Could you check a few things on this model? Use its own coordinates, in mm. A direction names the side the tool comes from. Coordinates: 2 decimals unless noted, no trailing zeros. Loops run counter-clockwise (first coordinate to the right, second up) from the corner with the lowest first, then second, coordinate; pieces in that order, holes last. Notation, with made-up numbers: M 64,54 L 120,54 A34 cw 120,90 Z; hole C 81.5,-9 d2. An arc over 180 degrees is marked long. Write each question's results on one line, items separated by ' | '.
Autodesk Fusion 360 part; units mm, degrees
sketch "main" plane through (0, 0, 0) normal (0, 0, 1) x (1, 0, 0)
  line L0 (-50, 15) -> (50, 15)
  line L1 (50, 15) -> (50, -15)
  line L2 (50, -15) -> (-50, -15)
  line L3 (-50, -15) -> (-50, 15)
  line L4 (-50, 15) -> (50, -15) construction
  line L5 (50, 15) -> (-50, -15) construction
  line L6 (30, 15) -> (-30, 15) construction
  line L7 (-30, 15) -> (-30, -15) construction
  line L8 (-30, -15) -> (30, -15) construction
  line L9 (30, -15) -> (30, 15) construction
  line L10 (-50, 15) -> (-30, -15) construction
  line L11 (-30, 15) -> (-50, -15) construction
  circle A0 centre (-40, 0) radius 2.75
  line L12 (30, 15) -> (50, -15) construction
  line L13 (50, 15) -> (30, -15) construction
  circle A1 centre (40, 0) radius 2.75
  line L14 (-50, -15) -> (50, -15)
  line L15 (50, -15) -> (50, -6.5)
  line L16 (50, -6.5) -> (-50, -6.5)
  line L17 (-50, -6.5) -> (-50, -15)
  line L18 (35.95, -4.05) -> (44.05, -4.05)
  line L19 (44.05, -4.05) -> (44.05, 4.05)
  line L20 (44.05, 4.05) -> (35.95, 4.05)
  line L21 (35.95, 4.05) -> (35.95, -4.05)
  line L22 (35.95, -4.05) -> (44.05, 4.05) construction
  line L23 (44.05, -4.05) -> (35.95, 4.05) construction
  line L24 (-44.05, -4.05) -> (-35.95, -4.05)
  line L25 (-35.95, -4.05) -> (-35.95, 4.05)
  line L26 (-35.95, 4.05) -> (-44.05, 4.05)
  line L27 (-44.05, 4.05) -> (-44.05, -4.05)
  line L28 (-44.05, -4.05) -> (-35.95, 4.05) construction
  line L29 (-35.95, -4.05) -> (-44.05, 4.05) construction
  line L30 (44.05, 4.05) -> (35.95, 4.05)
  line L31 (35.95, 4.05) -> (35.95, 15)
  line L32 (35.95, 15) -> (44.05, 15)
  line L33 (44.05, 15) -> (44.05, 4.05)
  line L34 (-35.95, 4.05) -> (-44.05, 4.05)
  line L35 (-44.05, 4.05) -> (-44.05, 15)
  line L36 (-44.05, 15) -> (-35.95, 15)
  line L37 (-35.95, 15) -> (-35.95, 4.05)
  point P0 (40, 0)
  point P1 (-40, 0)
  dimension "d1" = 100
  dimension "d2" = 30
  dimension "d3" = 60
  dimension "d4" = 30
  dimension "d5" = 5.5
  dimension "d6" = 5.5
  dimension "d7" = 100
  dimension "d8" = 8.5
  dimension "d17" = 8.1
  dimension "d18" = 8.1
  dimension "d19" = 8.1
  dimension "d20" = 8.1
  dimension "d21" = 8.1
  dimension "d22" = 10.95
  dimension "d23" = 8.1
  dimension "d24" = 10.95
extrude "Extrude1" add sketch "main" against normal blind 12
extrude "Extrude2" add sketch "main" against normal blind 22 from surface at -12 contours L1 L2 L3 L14 L15 L16 L17
extrude "Extrude3" add sketch "main" against normal blind 12 from surface at -34 contours L0 L1 L3 L16 L18 L19 L21 L24 L25 L27 L31 L33 L35 L37 | L0 L26 L34 L35 L36 L37 | L1 L2 L3 L14 L15 L16 L17 | L24 L25 L26 L27 L34 | L0 L20 L30 L31 L32 L33 | L18 L19 L20 L21 L30 | A0 | A1
extrude "Extrude4" cut sketch "main" along normal mid plane 3.7 from surface at -6 contours L0 L26 L34 L35 L36 L37 | L24 L25 L26 L27 L34 | L0 L20 L30 L31 L32 L33 | L18 L19 L20 L21 L30
equation "d5 = ( 2.75 * 2 ) * 1 mm"
equation "d14 = -22 mm - 12 mm"
(1) If we mould it in two halves opening along X, with no side actions, what happens to faces 1 (the flat face through (50, -10, -23)), 2 (the flat face through (-50, -7, -23)), 3 (the flat face through (-40, -4.05, -6)), 4 (the flat face through (-1, 4, -12))? For each: released by +X, released by -X, zero draft, split by the parting line, or undercut.
Reported:
face 1: released by +X | face 2: released by -X | face 3: undercut | face 4: zero draft
(2) Imagine slicing it at C-C, the plane z = -10. List the corners of the cut face in (x, y) for me.
Reported:
outline: M -50,-15 L 50,-15 L 50,15 L -50,15 Z; hole C -40,0 d5.5; hole C 40,0 d5.5
(3) Imagine slicing it at B-B, the plane x = -40. List the corners of the cut face in (y, z) for me.
Reported:
outline: M -15,-46 L 15,-46 L 15,-34 L -6.5,-34 L -6.5,-12 L -2.75,-12 L -2.75,-7.85 L -4.05,-7.85 L -4.05,-4.15 L -2.75,-4.15 L -2.75,0 L -15,0 Z; M 2.75,-12 L 15,-12 L 15,-7.85 L 2.75,-7.85 Z; M 2.75,-4.15 L 15,-4.15 L 15,0 L 2.75,0 Z
(4) Imagine slicing it at A-A, the plane y = 7.5. List the corners of the cut face in (x, z) for me, and give its area (3 significant figures).
Reported:
outline: M -50,-46 L 50,-46 L 50,-34 L -50,-34 Z; M -50,-12 L 50,-12 L 50,0 L -50,0 Z; hole M -44.05,-7.85 L -35.95,-7.85 L -35.95,-4.15 L -44.05,-4.15 Z; hole M 35.95,-7.85 L 44.05,-7.85 L 44.05,-4.15 L 35.95,-4.15 Z | area: 2,340 mm2
(5) Imagine slicing it at D-D, the plane y = 0. State how many separate pieces and enclosed holes the cut face has, and give its area (3 significant figures).
Reported:
separate pieces: 4 | enclosed holes: 0 | area: 2,250 mm2
(6) Will these pins go through, and if not, where does the flat tip stop? P1, Ø5, axis at x = 40, y = 0, coming from the +Z side; P2, Ø1, axis at x = 5.5, z = -17.5, coming from the +Y side.
Reported:
P1: stops at z = -34 | P2: stops at y = -6.5
(7) Please list where these lines run through material, in increasing order: probe 1 along Z at (x, y) = (-40, 4.25); probe 2 along Y at (x, z) = (40, -10.8); probe 3 along Z at (x, y) = (-25, -4.75). Write a range as from..to.
Reported:
probe 1: z = -46..-34, -12..-7.85, -4.15..0 | probe 2: y = -15..-2.75, 2.75..15 | probe 3: z = -46..-34, -12..0
(8) Which directions (+Z, -Z, +X, -X, +Y, -Y) give clear straight access to the entire face, cutting with the end or side of a thin tool? Please do faces 5 (the flat face through (-1, 15, -6)), 6 (the flat face through (-40, 6, -7.85)), 7 (the cylindrical face through (37.253, 0.121, -9.896)).
Reported:
face 5: +Z, -Z, +X, -X, +Y | face 6: +Y | face 7: +Z
